Can you work these out from the model? Positions are in its coordinate system, mm. Face numbers are marked on the shaded views. A direction names the side the tool comes from. Round coordinates to 2 decimals unless told otherwise and drop trailing zeros. Write each loop counter-clockwise with the first axis right and the second up, starting at its lowest first coordinate (ties: lowest second). Pieces come first, ordered by that corner, then holes. Notation, with made-up numbers: M 36,44.5 L 42,44.5 A15 ccw 42,65.5 Z; hole C -17,53 d9. An arc over 180 degrees is marked long. Answer in a Markdown table with one row per item. Add a question column.
(1) If we mould it in two halves opening along X, with no side actions, what happens to the marked faces 5 and 6? For each: released by +X, released by -X, zero draft, split by the parting line, or undercut.
(2) For the marked faces 1, 2, 3 and 4, which set-ups out of +Z, -Z, +X, -X, +Y, -Y let a thin tool reach every point of the face, with its end or its side?
(3) I'm going to push flat-ended pins straight in: pin 1 (1.9 mm diameter, centred on x = 42, z = 8.5, fed in from -Y); pin 2 (4 mm diameter, centred on x = 36.5, z = -24, fed in from +Y); pin 3 (2.5 mm diameter, centred on x = 24, z = -32.5, fed in from +Y); pin 4 (12 mm diameter, centred on x = -6, z = -23.5, fed in from +Y). Where does each tip first touch, or does it pass through?
(4) Suppose I cut it at C-C, the plane y = 6.25. Count the separate pieces of the cut face and the enclosed holes in it, then the cut area to 3 significant figures.
(5) Suppose I cut it at A-A, the plane y = 12.25. Write out the boundary of the cut face in (x, z), then the cut area to 3 significant figures.
(6) Suppose I cut it at B-B, the plane x = 0. Write out the boundary of the cut face in (y, z).
(7) If I drill on probe 1 along X at (y, z) = (11.5, 0); probe 2 along Z at (x, y) = (-14.5, 12); probe 3 along Z at (x, y) = (-12.5, 11), over which ranges is the centre line in solid material (lowest first)?
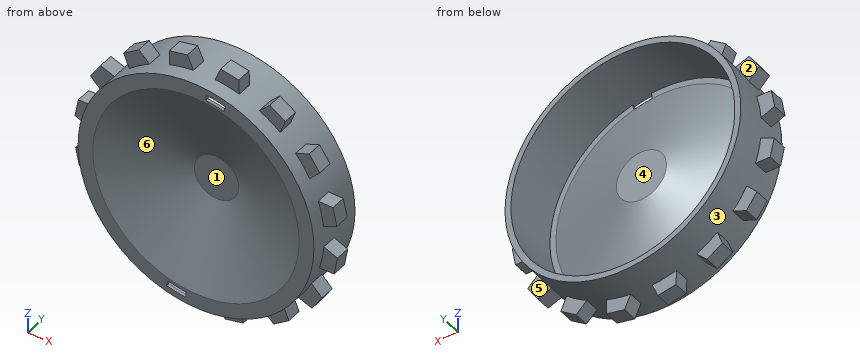
from build123d import *

# Parameters (mm, degrees)
SKETCH1_R           = 40
BOSS_EXTRUDE1_DEPTH = 10
SKETCH2_R           = 38
CUT_EXTRUDE1_DEPTH  = 9
CUT_EXTRUDE2_DEPTH  = 8
SKETCH4_R           = 36
BOSS_EXTRUDE2_DEPTH = 10
BOSS_EXTRUDE2_TAPER = 70
SKETCH5_R           = 35
CUT_EXTRUDE3_DEPTH  = 10
CUT_EXTRUDE3_DRAFT  = -70
BOSS_EXTRUDE4_START = -5
BOSS_EXTRUDE4_DEPTH = 5
BOSS_EXTRUDE5_START = 10
SKETCH8_R           = 40
SKETCH8_R_2         = 38
BOSS_EXTRUDE5_DEPTH = 10


with BuildPart() as part:
    # Sketch1 → Boss-Extrude1 (new body)
    with BuildSketch(Plane(origin=(0, 0, 0), x_dir=(1, 0, 0), z_dir=(0, 1, 0))):
        with Locations(Location((0, 0, 0), (0, 0, 270))):
            Circle(SKETCH1_R)
    extrude(amount=BOSS_EXTRUDE1_DEPTH)

    # Sketch2 → Cut-Extrude1 (cut)
    with BuildSketch(Plane(origin=(0, 10, 0), x_dir=(1, 0, 0), z_dir=(0, 1, 0))):
        with Locations(Location((0, 0, 0), (0, 0, 270))):
            Circle(SKETCH2_R)
    extrude(amount=-CUT_EXTRUDE1_DEPTH, mode=Mode.SUBTRACT)

    # Sketch3 → Cut-Extrude2 (cut)
    with BuildSketch(Plane(origin=(0, 1, 0), x_dir=(1, 0, 0), z_dir=(0, 1, 0))):
        with BuildLine():
            Line((-10.01806559, 36.655672983), (-9.49079898, 34.726427036))
            ThreePointArc((-9.49079898, 34.726427036), (-6.428076084, 35.421460132), (-3.316431646, 35.846914527))
            Line((-3.316431646, 35.846914527), (-3.500677849, 37.838409779))
            ThreePointArc((-3.500677849, 37.838409779), (-6.785191422, 37.389319028), (-10.01806559, 36.655672983))
        make_face()
        with BuildLine():
            Line((10.01806559, -36.655672983), (9.49079898, -34.726427036))
            ThreePointArc((9.49079898, -34.726427036), (6.428076084, -35.421460132), (3.316431646, -35.846914527))
            Line((3.316431646, -35.846914527), (3.500677849, -37.838409779))
            ThreePointArc((3.500677849, -37.838409779), (6.785191421, -37.389319028), (10.01806559, -36.655672983))
        make_face()
    extrude(amount=-CUT_EXTRUDE2_DEPTH, mode=Mode.SUBTRACT)

    # Sketch4 → Boss-Extrude2 (add)
    with BuildSketch(Plane(origin=(0, 1, 0), x_dir=(1, 0, 0), z_dir=(0, 1, 0))):
        Circle(SKETCH4_R)
    extrude(amount=BOSS_EXTRUDE2_DEPTH, taper=BOSS_EXTRUDE2_TAPER)


with BuildPart() as cut_extrude3_tool:
    # Sketch5 → Cut-Extrude3 (with draft: the straight prism first)
    with BuildSketch(Plane.XZ):
        Circle(SKETCH5_R)
    extrude(amount=-CUT_EXTRUDE3_DEPTH)
    # Cut-Extrude3: the draft: its side faces are tilted about the plane it starts from
    cut_extrude3_sides = [cut_extrude3_tool.faces().sort_by_distance(p)[0] for p in [
        (-35, 5, 0),
    ]]
    draft(cut_extrude3_sides, Plane.XZ, CUT_EXTRUDE3_DRAFT)


with BuildPart() as part_1:
    add(part.part)

    # Cut-Extrude3: cut by cut_extrude3_tool
    add(cut_extrude3_tool.part, mode=Mode.SUBTRACT)

    # Sketch7 → Boss-Extrude4 (add)
    with BuildSketch(Plane(origin=(0, 10, 0), x_dir=(1, 0, 0), z_dir=(0, 1, 0)).offset(BOSS_EXTRUDE4_START)):
        with BuildLine():
            Line((-11.051326445, 43.40114745), (-11.217125783, 38.395000836))
            ThreePointArc((-11.217125783, 38.395000836), (-7.142306759, 39.357177924), (-2.989235129, 39.888149535))
            Line((-2.989235129, 39.888149535), (-4.90350342, 44.516817838))
            Line((-4.90350342, 44.516817838), (-11.051326445, 43.40114745))
        make_face()
        with BuildLine():
            Line((6.398805765, 44.326591353), (4.329857781, 39.764963619))
            ThreePointArc((4.329857781, 39.764963619), (8.462708906, 39.094533607), (12.502840822, 37.995775705))
            Line((12.502840822, 37.995775705), (12.505602201, 43.004666372))
            Line((12.505602201, 43.004666372), (6.398805765, 44.326591353))
        make_face()
        with BuildLine():
            Line((22.874777803, 38.503713544), (19.217659748, 35.081071161))
            ThreePointArc((19.217659748, 35.081071161), (22.779353856, 32.880100941), (26.091472595, 30.318889455))
            Line((26.091472595, 30.318889455), (28.01084325, 34.94544429))
            Line((28.01084325, 34.94544429), (22.874777803, 38.503713544))
        make_face()
        with BuildLine():
            Line((35.868272281, 26.818994385), (31.179747227, 25.05640363))
            ThreePointArc((31.179747227, 25.05640363), (33.628048676, 21.659970966), (35.707914186, 18.026227128))
            Line((35.707914186, 18.026227128), (39.251687333, 21.566095096))
            Line((39.251687333, 21.566095096), (35.868272281, 26.818994385))
        make_face()
        with BuildLine():
            Line((43.40114745, 11.051326445), (38.395000836, 11.217125783))
            ThreePointArc((38.395000836, 11.217125783), (39.357177924, 7.142306759), (39.888149535, 2.989235129))
            Line((39.888149535, 2.989235129), (44.516817838, 4.90350342))
            Line((44.516817838, 4.90350342), (43.40114745, 11.051326445))
        make_face()
        with BuildLine():
            Line((44.326591353, -6.398805765), (39.764963619, -4.329857781))
            ThreePointArc((39.764963619, -4.329857781), (39.094533607, -8.462708906), (37.995775705, -12.502840822))
            Line((37.995775705, -12.502840822), (43.004666372, -12.505602201))
            Line((43.004666372, -12.505602201), (44.326591353, -6.398805765))
        make_face()
        with BuildLine():
            Line((38.503713544, -22.874777803), (35.081071161, -19.217659748))
            ThreePointArc((35.081071161, -19.217659748), (32.880100941, -22.779353856), (30.318889455, -26.091472595))
            Line((30.318889455, -26.091472595), (34.94544429, -28.01084325))
            Line((34.94544429, -28.01084325), (38.503713544, -22.874777803))
        make_face()
        with BuildLine():
            Line((26.818994385, -35.868272281), (25.05640363, -31.179747227))
            ThreePointArc((25.05640363, -31.179747227), (21.659970966, -33.628048676), (18.026227128, -35.707914186))
            Line((18.026227128, -35.707914186), (21.566095096, -39.251687333))
            Line((21.566095096, -39.251687333), (26.818994385, -35.868272281))
        make_face()
        with BuildLine():
            Line((11.051326445, -43.40114745), (11.217125783, -38.395000836))
            ThreePointArc((11.217125783, -38.395000836), (7.142306759, -39.357177924), (2.989235129, -39.888149535))
            Line((2.989235129, -39.888149535), (4.90350342, -44.516817838))
            Line((4.90350342, -44.516817838), (11.051326445, -43.40114745))
        make_face()
        with BuildLine():
            Line((-6.398805765, -44.326591353), (-4.329857781, -39.764963619))
            ThreePointArc((-4.329857781, -39.764963619), (-8.462708906, -39.094533607), (-12.502840822, -37.995775705))
            Line((-12.502840822, -37.995775705), (-12.505602201, -43.004666372))
            Line((-12.505602201, -43.004666372), (-6.398805765, -44.326591353))
        make_face()
        with BuildLine():
            Line((-22.874777803, -38.503713544), (-19.217659748, -35.081071161))
            ThreePointArc((-19.217659748, -35.081071161), (-22.779353856, -32.880100941), (-26.091472595, -30.318889455))
            Line((-26.091472595, -30.318889455), (-28.01084325, -34.94544429))
            Line((-28.01084325, -34.94544429), (-22.874777803, -38.503713544))
        make_face()
        with BuildLine():
            Line((-35.868272281, -26.818994385), (-31.179747227, -25.05640363))
            ThreePointArc((-31.179747227, -25.05640363), (-33.628048676, -21.659970966), (-35.707914186, -18.026227128))
            Line((-35.707914186, -18.026227128), (-39.251687333, -21.566095096))
            Line((-39.251687333, -21.566095096), (-35.868272281, -26.818994385))
        make_face()
        with BuildLine():
            Line((-43.40114745, -11.051326445), (-38.395000836, -11.217125783))
            ThreePointArc((-38.395000836, -11.217125783), (-39.357177924, -7.142306759), (-39.888149535, -2.989235129))
            Line((-39.888149535, -2.989235129), (-44.516817838, -4.90350342))
            Line((-44.516817838, -4.90350342), (-43.40114745, -11.051326445))
        make_face()
        with BuildLine():
            Line((-44.326591353, 6.398805765), (-39.764963619, 4.329857781))
            ThreePointArc((-39.764963619, 4.329857781), (-39.094533607, 8.462708906), (-37.995775705, 12.502840822))
            Line((-37.995775705, 12.502840822), (-43.004666372, 12.505602201))
            Line((-43.004666372, 12.505602201), (-44.326591353, 6.398805765))
        make_face()
        with BuildLine():
            Line((-38.503713544, 22.874777803), (-35.081071161, 19.217659748))
            ThreePointArc((-35.081071161, 19.217659748), (-32.880100941, 22.779353856), (-30.318889455, 26.091472595))
            Line((-30.318889455, 26.091472595), (-34.94544429, 28.01084325))
            Line((-34.94544429, 28.01084325), (-38.503713544, 22.874777803))
        make_face()
        with BuildLine():
            Line((-26.818994385, 35.868272281), (-25.05640363, 31.179747227))
            ThreePointArc((-25.05640363, 31.179747227), (-21.659970966, 33.628048676), (-18.026227128, 35.707914186))
            Line((-18.026227128, 35.707914186), (-21.566095096, 39.251687333))
            Line((-21.566095096, 39.251687333), (-26.818994385, 35.868272281))
        make_face()
    extrude(amount=BOSS_EXTRUDE4_DEPTH)

    # Sketch8 → Boss-Extrude5 (add)
    with BuildSketch(Plane(origin=(0, 10, 0), x_dir=(1, 0, 0), z_dir=(0, 1, 0)).offset(BOSS_EXTRUDE5_START)):
        with Locations(Location((0, 0, 0), (0, 0, 270))):
            Circle(SKETCH8_R)
        with Locations(Location((0, 0, 0), (0, 0, 270))):
            Circle(SKETCH8_R_2, mode=Mode.SUBTRACT)
    extrude(amount=-BOSS_EXTRUDE5_DEPTH)


solid = part_1.part
Calculated:
| question | item | result |
|---|---|---|
| 1 | face 5 | zero draft |
| 1 | face 6 | undercut |
| 2 | face 1 | -Y |
| 2 | face 2 | +Z, -X, +Y |
| 2 | face 3 | none |
| 2 | face 4 | +Y |
| 3 | pin 1 | y = 5 |
| 3 | pin 2 | y = 10 |
| 3 | pin 3 | y = 20 |
| 3 | pin 4 | y = 7.46 |
| 4 | separate pieces | 2 |
| 4 | enclosed holes | 2 |
| 4 | area | 1,510 mm² |
| 5 | outline | C 0,0 d80; hole C 0,0 d76 |
| 5 | area | 490 mm² |
| 6 | outline | M 0,-40 L 20,-40 L 20,-38 L 1,-38 L 1,-36 L 11,-8.53 L 11,8.53 L 1,36 L 1,38 L 20,38 L 20,40 L 0,40 L 0,35 L 10,7.53 L 10,-7.53 L 0,-35 Z |
| 7 | probe 1 | -40 to -38, 38 to 40 |
| 7 | probe 2 | -37.28 to -35.12, 35.12 to 37.28 |
| 7 | probe 3 | -38 to -35.89, 35.89 to 38 |
